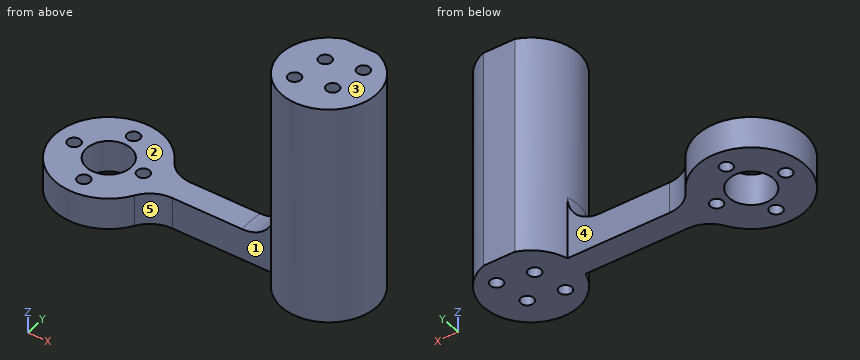
from build123d import *

# Parameters (mm, degrees)
SKETCH1_R           = 1.9999999999999996
SKETCH1_R_2         = 2
SKETCH1_R_3         = 7
SKETCH1_R_4         = 1.9999999999999967
BOSS_EXTRUDE1_DEPTH = 10
SKETCH2_R           = 15.000000000000057
SKETCH2_R_2         = 1.9999999999999967
BOSS_EXTRUDE2_DEPTH = 60
CUT_EXTRUDE1_DEPTH  = 112.41813137905342
FILLET1_R           = 10
FILLET2_R           = 10


with BuildPart() as part:
    # Sketch1 → Boss-Extrude1 (new body)
    with BuildSketch(Plane.XY):
        with BuildLine():
            Line((55.54316770519905, 4), (16.522711641858304, 4))
            ThreePointArc((16.522711641858304, 4), (-17, -5.47e-15), (16.522711641858304, -3.9999999999999996))
            Line((16.522711641858304, -4), (55.54316770519905, -4))
            ThreePointArc((55.54316770519898, -4.000000000000017), (85.00000000000006, 0), (55.54316770519898, 4.0000000000000195))
        make_face()
        with Locations((11, 1.73e-15)):
            Circle(SKETCH1_R, mode=Mode.SUBTRACT)
        with Locations((0, 11)):
            Circle(SKETCH1_R_2, mode=Mode.SUBTRACT)
        with Locations((8.7e-16, -11)):
            Circle(SKETCH1_R_2, mode=Mode.SUBTRACT)
        with Locations((-11, -2.6e-15)):
            Circle(SKETCH1_R, mode=Mode.SUBTRACT)
        Circle(SKETCH1_R_3, mode=Mode.SUBTRACT)
        with Locations((76.36396103067892, 6.363961030678928)):
            Circle(SKETCH1_R_4, mode=Mode.SUBTRACT)
        with Locations((63.636038969321085, -6.363961030678926)):
            Circle(SKETCH1_R_4, mode=Mode.SUBTRACT)
        with Locations((74.24264068711929, -4.242640687119276)):
            Circle(SKETCH1_R_4, mode=Mode.SUBTRACT)
        with Locations((65.75735931288074, 4.242640687119292)):
            Circle(SKETCH1_R_4, mode=Mode.SUBTRACT)
    extrude(amount=BOSS_EXTRUDE1_DEPTH)

    # Sketch2 → Boss-Extrude2 (add)
    with BuildSketch(Plane.XY.offset(10)):
        with Locations(Location((70, 0, 0), (0, 0, 164.533990047))):
            Circle(SKETCH2_R)
        with Locations((63.636038969321085, -6.363961030678926)):
            Circle(SKETCH2_R_2, mode=Mode.SUBTRACT)
        with Locations((74.24264068711929, -4.242640687119276)):
            Circle(SKETCH2_R_2, mode=Mode.SUBTRACT)
        with Locations((76.36396103067892, 6.363961030678928)):
            Circle(SKETCH2_R_2, mode=Mode.SUBTRACT)
        with Locations((65.75735931288074, 4.242640687119292)):
            Circle(SKETCH2_R_2, mode=Mode.SUBTRACT)
    extrude(amount=BOSS_EXTRUDE2_DEPTH)

    # Sketch3 → Cut-Extrude1 (cut, through all)
    with BuildSketch(Plane.XY.offset(69.99999999999999)):
        with BuildLine():
            ThreePointArc((74.99999999999999, 14.142135623731015), (70, 15.000000000000057), (65, 14.142135623731011))
            Line((65, 14.142135623731008), (74.99999999999999, 14.142135623731008))
        make_face()
    extrude(amount=-CUT_EXTRUDE1_DEPTH, mode=Mode.SUBTRACT)

    # Fillet1
    fillet1_edges = [part.edges().sort_by_distance(p)[0] for p in [
        (54.99999999999994, -5.50493e-11, 10),
    ]]
    fillet(fillet1_edges, radius=FILLET1_R)

    # Fillet2
    fillet2_edges = [part.edges().sort_by_distance(p)[0] for p in [
        (16.522711641858304, 4, 5),
        (16.522711641858308, -4.000000000000004, 5),
    ]]
    fillet(fillet2_edges, radius=FILLET2_R)


solid = part.part
The listing builds one solid part. Answer for the finished solid, in the listing's coordinates (mm). Face numbers are marked on the shaded views. A direction names the side the tool comes from. Give positions to 0.01 mm unless a question says otherwise; leave off trailing zeros. Order: outer loops, then holes, each group sorted by start corner. A loop starts at its lowest first (then second) coordinate and runs counter-clockwise, first axis right, second up. Notation, with made-up numbers: (15.5, 33) - (28.5, 33) arc R31 ccw to (28.5, 65) - close; hole circle Ø9 at (41, 29.25). An arc over 180 degrees is marked (long way). Answer as CSV lines item,"result".
Q1. Determine the mould class of the marked faces 1 and 2 for opening direction X: pulls with the +X half, pulls with the -X half, needs draft (parallel to the pull), parting line crosses it, or undercut.
Answer key:
face 1,"undercut"
face 2,"needs draft"
Q2. Each of these flat-tipped pins is pushed along its axis until it touches: pin 1 Ø5 at (x, y) = (11, -3.5) entering from +Z; pin 2 Ø3 at (x, z) = (67.5, 19) entering from +Y; pin 3 Ø12 at (y, z) = (-7, 10) entering from +X. Where does it stop, or does it pass through?
Answer key:
pin 1,"stops at z = 10"
pin 2,"stops at y = 14.14"
pin 3,"stops at x = 84.97"
Q3. A cutting plane is placed at D-D, the plane z = 12. Determine the outline of the cut face in (x, y), and give its area (3 significant figures).
Answer key:
outline,"(51.43, -4) - (55.54, -4) arc R15 ccw (long way) to (75, 14.14) - (65, 14.14) arc R15 ccw to (55.54, 4) - (51.43, 4) arc R19 ccw to start; hole circle Ø4 at (63.64, -6.36); hole circle Ø4 at (65.76, 4.24); hole circle Ø4 at (74.24, -4.24); hole circle Ø4 at (76.36, 6.36)"
area,"683 mm^2"
Q4. A cutting plane is placed at A-A, the plane y = 0. Determine the outline of the cut face in (x, z).
Answer key:
outline,"(-17, 0) - (-13, 0) - (-13, 10) - (-17, 10) - close; (-9, 0) - (-7, 0) - (-7, 10) - (-9, 10) - close; (7, 0) - (9, 0) - (9, 10) - (7, 10) - close; (13, 0) - (85, 0) - (85, 70) - (55, 70) - (55, 20) arc R10 cw to (45, 10) - (13, 10) - close"
Q5. Straight lines are drawn through the part: L1, parallel to Y at x = 75, z = 26.5; L2, parallel to Y at x = 64, z = 39; L3, parallel to Z at x = -1, y = 13. For each, find the intervals that lie inside material, in ascending order.
Answer key:
L1,"y = -14.14 to -6.09, -2.39 to 4.9, 7.83 to 14.14"
L2,"y = -13.75 to -8.33, -4.4 to 3.29, 5.2 to 13.75"
L3,"z = 0 to 10"
Q6. A cutting plane is placed at B-B, the plane x = 0. Determine the outline of the cut face in (y, z).
Answer key:
outline,"(-17, 0) - (-13, 0) - (-13, 10) - (-17, 10) - close; (-9, 0) - (-7, 0) - (-7, 10) - (-9, 10) - close; (7, 0) - (9, 0) - (9, 10) - (7, 10) - close; (13, 0) - (17, 0) - (17, 10) - (13, 10) - close"
Q7. A cutting plane is placed at C-C, the plane x = -11. Determine the outline of the cut face in (y, z), and give its area (3 significant figures).
Answer key:
outline,"(-12.96, 0) - (-2, 0) - (-2, 10) - (-12.96, 10) - close; (2, 0) - (12.96, 0) - (12.96, 10) - (2, 10) - close"
area,"219 mm^2"
Q8. Which of the six approach directions +Z, -Z, +X, -X, +Y, -Y give full straight-line access (tool end or side, diameter ignored) to the marked faces 3, 4 and 5?
Answer key:
face 3,"+Z, +X, -X, +Y, -Y"
face 4,"+Z, -Z, +Y"
face 5,"+Z, -Z, -Y"
